Geometry: final body of the model. Coordinates: model frame, mm. Round coordinates to 2 decimals unless told otherwise and drop trailing zeros. Write each loop counter-clockwise with the first axis right and the second up, starting at its lowest first coordinate (ties: lowest second). Pieces come first, ordered by that corner, then holes. Notation, with made-up numbers: M 74.25,7.5 L 91.25,7.5 A21 cw 91.25,16.5 Z; hole C 83,57 d3. An arc over 180 degrees is marked long. Use one line per item in the form item = value. Start each with the question number.
Item 1: Pin query (flat end, axial travel): pin 1 Ø12 at (x, y) = (0, 0) entering from -Z; pin 2 Ø4 at (y, z) = (60.5, 2.5) entering from -X; pin 3 Ø5 at (x, z) = (-55, 4) entering from -Y; pin 4 Ø5 at (y, z) = (-7.5, 5.5) entering from +X. Return the tip coordinate at first contact, or that it passes through.
Item 2: Section query C-C (x = -79.5). Return loops of the section in (y, z).
Item 3: Ray query, probe 1 along Y at (x, z) = (0, 6.25); probe 2 along X at (y, z) = (0.5, 8.25); probe 3 along X at (y, z) = (-3.5, 5.5). Return the intervals inside material, ascending.
Item 4: Section query B-B (z = 3.75). Return loops of the section in (x, y), and give its area (3 significant figures).
Item 5: Section query D-D (x = 0). Return loops of the section in (y, z).
Item 6: Section query A-A (y = 0). Return loops of the section in (x, z), and give its area (3 significant figures).
from build123d import *

# Parameters (mm, degrees)
SKETCH_R      = 10
EXTRUDE_DEPTH = 10


with BuildPart() as part:
    # Sketch → Extrude (new body)
    with BuildSketch(Plane.XY):
        with BuildLine():
            ThreePointArc((-10, -38.729833), (0, -40), (10, -38.729833))
            Line((85, -19.364917), (10, -38.729833))
            ThreePointArc((85, -19.364917), (99.294714, -5.264411), (94.142136, 14.142136))
            Line((14.142136, 94.142136), (94.142136, 14.142136))
            ThreePointArc((14.142136, 94.142136), (0, 100), (-14.142136, 94.142136))
            Line((-94.142136, 14.142136), (-14.142136, 94.142136))
            ThreePointArc((-94.142136, 14.142136), (-99.294714, -5.264411), (-85, -19.364917))
            Line((-10, -38.729833), (-85, -19.364917))
        make_face()
        Circle(SKETCH_R, mode=Mode.SUBTRACT)
        with Locations((-80, 0)):
            Circle(SKETCH_R, mode=Mode.SUBTRACT)
        with Locations((80, 0)):
            Circle(SKETCH_R, mode=Mode.SUBTRACT)
        with Locations((0, 80)):
            Circle(SKETCH_R, mode=Mode.SUBTRACT)
    extrude(amount=EXTRUDE_DEPTH)


solid = part.part
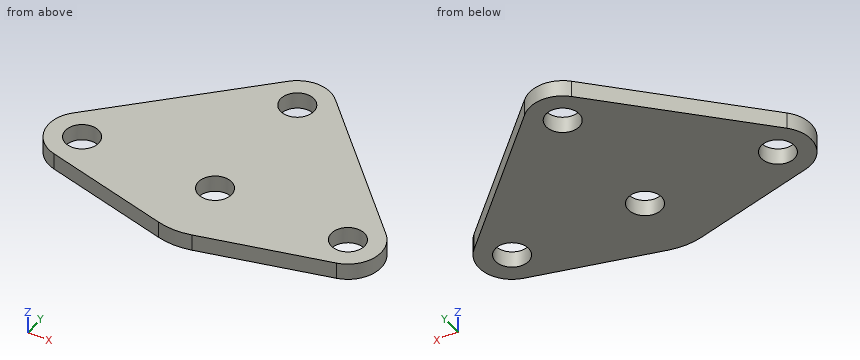
Working result:
q1.pin_1 = through
q1.pin_2 = -49.78
q1.pin_3 = -27.76
q1.pin_4 = 99.36
q2.outline = M -20.79,0 L -9.99,0 L -9.99,10 L -20.79,10 Z; M 9.99,0 L 28.78,0 L 28.78,10 L 9.99,10 Z
q3.probe_1 = -40 to -10, 10 to 70, 90 to 100
q3.probe_2 = -99.99 to -89.99, -70.01 to -9.99, 9.99 to 70.01, 89.99 to 99.99
q3.probe_3 = -99.69 to -89.37, -70.63 to -9.37, 9.37 to 70.63, 89.37 to 99.69
q4.outline = M -94.14,14.14 A20 ccw -85,-19.36 L -10,-38.73 A40 ccw 10,-38.73 L 85,-19.36 A20 ccw 94.14,14.14 L 14.14,94.14 A20 ccw -14.14,94.14 Z; hole C -80,0 d20; hole C 0,0 d20; hole C 0,80 d20; hole C 80,0 d20
q4.area = 15,900 mm²
q5.outline = M -40,0 L -10,0 L -10,10 L -40,10 Z; M 10,0 L 70,0 L 70,10 L 10,10 Z; M 90,0 L 100,0 L 100,10 L 90,10 Z
q6.outline = M -100,0 L -90,0 L -90,10 L -100,10 Z; M -70,0 L -10,0 L -10,10 L -70,10 Z; M 10,0 L 70,0 L 70,10 L 10,10 Z; M 90,0 L 100,0 L 100,10 L 90,10 Z
q6.area = 1,400 mm²
